Can you work these out from the model? Positions are in its coordinate system, mm. Coordinates: 2 decimals unless noted, no trailing zeros. Loops run counter-clockwise (first coordinate to the right, second up) from the corner with the lowest first, then second, coordinate; pieces in that order, holes last.
```python
from build123d import *

# Parameters (mm, degrees)
F0_R     = 2.65378
F0_R_2   = 2.705133
F1_DEPTH = 3.175


with BuildPart() as f1:
    # F0 (on Top) → F1 (new body)
    with BuildSketch(Plane.XY):
        Polygon((0, 7.664707), (0, 0), (19.709434, 0), (22.774175, 18.209429), (28.829604, 20.252014), (28.829604, 25.431277), (16.022975, 25.431277), align=None)
        with Locations((5.134751, 4.33671)):
            Circle(F0_R, mode=Mode.SUBTRACT)
        with Locations((12.520132, 4.268356)):
            Circle(F0_R_2, mode=Mode.SUBTRACT)
    extrude(amount=F1_DEPTH)


solid = f1.part
```
Item 1: Suppose I cut it at A-A, the plane x = 3. Please give me the cut outline in (y, z) (3 decimals), plus the area to 3 significant figures.
Results are:
outline: (0, 0) - (2.76, 0) - (2.76, 3.175) - (0, 3.175) - close; (5.913, 0) - (10.991, 0) - (10.991, 3.175) - (5.913, 3.175) - close
area: 24.9 mm2
Item 2: I need wall thicknesses on line 1 along X through (y, z) = (6.25, 0.25); line 2 along X through (y, z) = (3.5, 1.7); line 3 along Y through (x, z) = (13.75, 1.1). Which ranges of each line are inside material? Lowest first, please.
Results are:
line 1: x = 0 to 3.3, 6.97 to 10.68, 14.36 to 20.76
line 2: x = 0 to 2.62, 7.65 to 9.93, 15.11 to 20.3
line 3: y = 0 to 1.86, 6.68 to 22.91
Item 3: Suppose I cut it at B-B, the plane y = 3.25. Please give me the cut outline in (x, z) (3 decimals), plus the area to 3 significant figures.
Results are:
outline: (0, 0) - (2.714, 0) - (2.714, 3.175) - (0, 3.175) - close; (7.556, 0) - (10.014, 0) - (10.014, 3.175) - (7.556, 3.175) - close; (15.026, 0) - (20.256, 0) - (20.256, 3.175) - (15.026, 3.175) - close
area: 33.0 mm2
Item 4: Suppose I cut it at C-C, the plane z = 1.35. Please give me the cut outline in (x, y).
Results are:
outline: (0, 0) - (19.71, 0) - (22.77, 18.21) - (28.83, 20.25) - (28.83, 25.43) - (16.02, 25.43) - (0, 7.66) - close; hole circle Ø5.31 at (5.13, 4.34); hole circle Ø5.41 at (12.52, 4.27)
Item 5: Suppose I cut it at D-D, the plane x = 14.5. Please give me the cut outline in (y, z) (3 decimals).
Results are:
outline: (0, 0) - (2.425, 0) - (2.425, 3.175) - (0, 3.175) - close; (6.112, 0) - (23.743, 0) - (23.743, 3.175) - (6.112, 3.175) - close
Item 6: I'm going to push a flat-ended pin straight in: P1, Ø1.5, axis at y = 15, z = 1, coming from the -X side. Where does the tip first touch, or does it pass through?
Results are:
P1: stops at x = 5.94
Item 7: We'd pull the mould along Y, two halves only. Please class faces 1 (the face through (28.83, 23, 2)), 2 (the face through (23, 25.431, 2)), 3 (the face through (4.559, 1.746, 1.565)): +Y half, -Y half, draft (parallel to the pull), parting line (faces both ways), or undercut.
Results are:
face 1: draft
face 2: +Y half
face 3: undercut
